Geometry check sheet. Reference: drawing and pictorial views, mm from the part's lowest x, y, z. Round coordinates to 2 decimals unless told otherwise and drop trailing zeros. Loops run counter-clockwise (first coordinate to the right, second up) from the corner with the lowest first, then second, coordinate; pieces in that order, holes last. Notation, with made-up numbers: (77, -26) - (89, -26) arc R20 cw to (89, 1) - close; hole circle Ø1 at (55, 59). An arc over 180 degrees is marked (long way). Return JSON: item names as keys, results as strings.
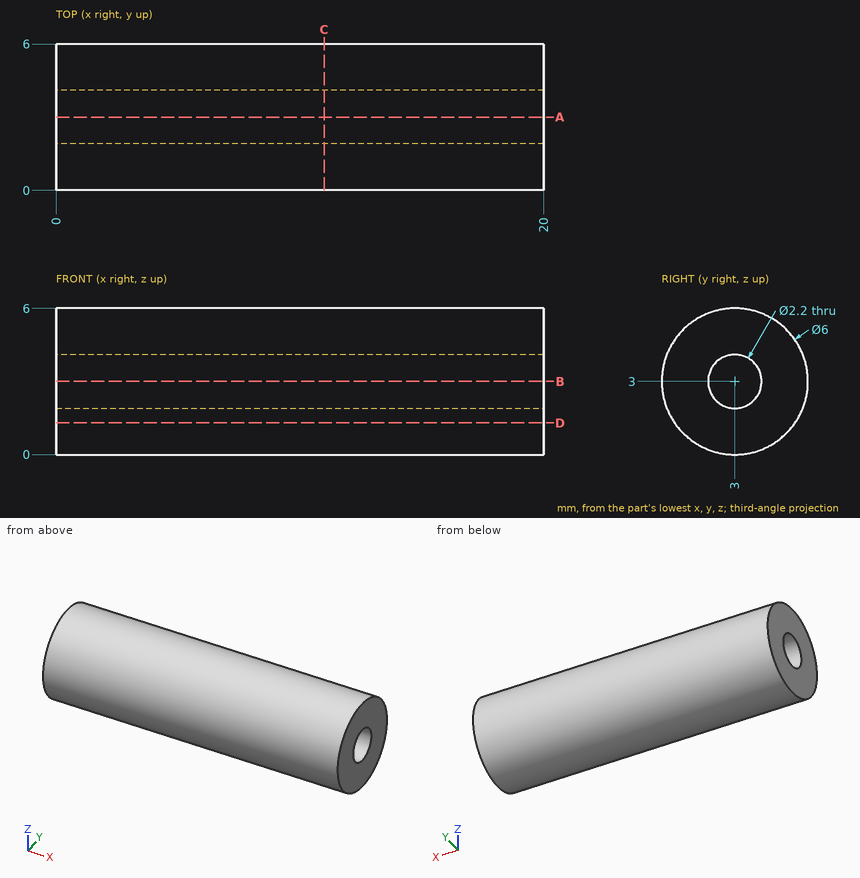
Q1. Scan lines: probe 1 along Y at (x, z) = (11.75, 3); probe 2 along Z at (x, y) = (12.5, 3.55). Record each from-to range of solid material in increasing order. Write a range as [from, to].
Answer key:
{"probe 1": "y = [0, 1.9], [4.1, 6]", "probe 2": "z = [0.05, 2.05], [3.95, 5.95]"}
Q2. Sectioned sample at C-C (x = 11). Enter the section's corners in (y, z), plus the area to 3 significant figures.
Answer key:
{"outline": "circle Ø6 at (3, 3); hole circle Ø2.2 at (3, 3)", "area": "24.5 mm²"}
Q3. Depth check by flat-ended pin: P1, Ø1.5, axis at y = 0.5, z = 2, coming from the -X side. Enter the tip coordinate at first touch or a pass-through.
Answer key:
{"P1": "stops at x = 0"}
Q4. Sectioned sample at A-A (y = 3). Enter the section's corners in (x, z), plus the area to 3 significant figures.
Answer key:
{"outline": "(0, 0) - (20, 0) - (20, 1.9) - (0, 1.9) - close; (0, 4.1) - (20, 4.1) - (20, 6) - (0, 6) - close", "area": "76.0 mm²"}
Q5. Sectioned sample at D-D (z = 1.3). Enter the section's corners in (x, y), plus the area to 3 significant figures.
Answer key:
{"outline": "(0, 0.53) - (20, 0.53) - (20, 5.47) - (0, 5.47) - close", "area": "98.9 mm²"}
